Part model, mm, in its own coordinate system. Face numbers are marked on the shaded views. A direction names the side the tool comes from. Coordinates: 2 decimals unless noted, no trailing zeros. Loops run counter-clockwise (first coordinate to the right, second up) from the corner with the lowest first, then second, coordinate; pieces in that order, holes last. Notation, with made-up numbers: (-7.5, 31) -> (28.5, 31) arc R20 ccw to (28.5, 54) -> close; hole circle Ø10 at (-27, 83.5). An arc over 180 degrees is marked (long way). One line per question, with ' | ' between items. Start each with the question number.
1) Cut at C-C (y = 66.5). List the corners of the cut face in (x, z), plus the area to 3 significant figures.
2) Probe L1, parallel to X at y = 10, z = 38.5; L2, parallel to Y at x = 61, z = -28.5; L3, parallel to X at y = 67, z = -42.5. List the from-to ranges inside material, lowest first. Write a range as from..to.
3) 3-axis set-ups, long thin cutter, end or side, ignore diameter. For the marked faces 1 and 2: which of +Z, -Z, +X, -X, +Y, -Y reach the whole face in a straight line?
4) Drop flat-ended pins along their axis: pin 1 (1.2 mm diameter, centred on x = 79.45, z = -62.77, fed in from -Y); pin 2 (2 mm diameter, centred on x = 28, z = 47, fed in from -Y). Give the stop position or say it passes through.
5) Two-plate mould, pull along X, no slides. Class the marked faces 3, 4 and 5: released by +X, released by -X, zero draft, split by the parting line, or undercut.
6) Cut at A-A (y = 29.5). List the corners of the cut face in (x, z), plus the area to 3 significant figures.
7) Cut at B-B (z = -47). List the corners of the cut face in (x, y), plus the area to 4 significant figures.
8) Cut at D-D (x = 65). List the corners of the cut face in (y, z).
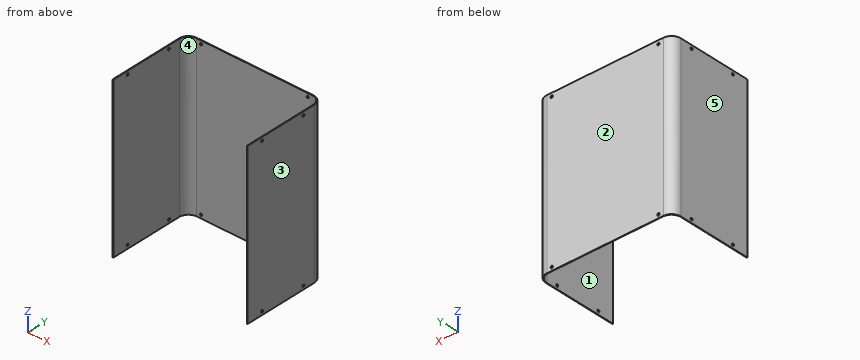
from build123d import *

# Parameters (mm, degrees)
SKETCH_1_W          = 117
SKETCH_1_H          = 138
EXTRUDE_1_DEPTH     = 72.5
CUT_EXTRUDE_1_DEPTH = 140
CUT_EXTRUDE_2_DEPTH = 140
SKETCH_6_R          = 1
CUT_EXTRUDE_5_DEPTH = 140
SKETCH_7_R          = 1
CUT_EXTRUDE_7_DEPTH = 140


with BuildPart() as part:
    # Эскиз1 → Бобышка-Вытянуть1 (new body)
    with BuildSketch(Plane(origin=(0, 0, 0), x_dir=(1, 0, 0), z_dir=(0, 1, 0))):
        with Locations((33.234281685, -3.234040823)):
            Rectangle(SKETCH_1_W, SKETCH_1_H)
    extrude(amount=EXTRUDE_1_DEPTH)

    # Эскиз2 → Вырез-Вытянуть1 (cut)
    with BuildSketch(Plane(origin=(0, 0, -65.765959177), x_dir=(-1, 0, 0), z_dir=(0, 0, -1))):
        with BuildLine():
            Line((-91.734281685, 64.5), (-91.734281685, 72.5))
            Line((-91.734281685, 72.5), (-83.734281685, 72.5))
            ThreePointArc((-83.734281685, 72.5), (-89.391135935, 70.156854249), (-91.734281685, 64.5))
        make_face()
        with BuildLine():
            Line((17.265718315, 72.5), (25.265718315, 72.5))
            Line((25.265718315, 72.5), (25.265718315, 64.5))
            ThreePointArc((25.265718315, 64.5), (22.922572564, 70.156854249), (17.265718315, 72.5))
        make_face()
    extrude(amount=-CUT_EXTRUDE_1_DEPTH, mode=Mode.SUBTRACT)

    # Эскиз3 → Вырез-Вытянуть2 (cut)
    with BuildSketch(Plane.XY.offset(72.234040823)):
        with BuildLine():
            Line((-24.765718315, 0), (91.234281685, 0))
            Line((91.234281685, 0), (91.234281685, 64))
            ThreePointArc((91.234281685, 64), (88.891135935, 69.656854249), (83.234281685, 72))
            Line((83.234281685, 72), (-16.765718315, 72))
            ThreePointArc((-16.765718315, 72), (-22.422572564, 69.656854249), (-24.765718315, 64))
            Line((-24.765718315, 64), (-24.765718315, 0))
        make_face()
    extrude(amount=-CUT_EXTRUDE_2_DEPTH, mode=Mode.SUBTRACT)

    # Эскиз6 → Вырез-Вытянуть5 (cut)
    with BuildSketch(Plane.ZY.offset(25.265718315)):
        with Locations((-62.765959177, 14)):
            Circle(SKETCH_6_R)
        with Locations(Location((69.234040823, 14, 0), (0, 0, 270))):
            Circle(SKETCH_6_R)
        with Locations((-62.765959177, 54)):
            Circle(SKETCH_6_R)
        with Locations(Location((69.234040823, 54, 0), (0, 0, 270))):
            Circle(SKETCH_6_R)
    extrude(amount=-CUT_EXTRUDE_5_DEPTH, mode=Mode.SUBTRACT)

    # Эскиз7 → Вырез-Вытянуть7 (cut)
    with BuildSketch(Plane(origin=(0, 72, 0), x_dir=(-1, 0, 0), z_dir=(0, -1, 0))):
        with Locations(Location((-79.454291209, 62.765959177, 0), (0, 0, 90))):
            Circle(SKETCH_7_R)
        with Locations((-582.904668668, 16.142688411)):
            Circle(SKETCH_7_R)
        with Locations(Location((12.9857274, -69.234040823, 0), (0, 0, 90))):
            Circle(SKETCH_7_R)
        with Locations(Location((-79.454291209, -69.234040823, 0), (0, 0, 90))):
            Circle(SKETCH_7_R)
        with Locations(Location((12.985727838, 62.765959177, 0), (0, 0, 90))):
            Circle(SKETCH_7_R)
    extrude(amount=-CUT_EXTRUDE_7_DEPTH, mode=Mode.SUBTRACT)


solid = part.part
Reported:
1) outline: (-25.01, -65.77) -> (-24.37, -65.77) -> (-24.37, 72.23) -> (-25.01, 72.23) -> close; (90.83, -65.77) -> (91.48, -65.77) -> (91.48, 72.23) -> (90.83, 72.23) -> close | area: 178 mm²
2) L1: x = -25.27..-24.77, 91.23..91.73 | L2: y = 72..72.5 | L3: x = -24.87..-24.18, 90.65..91.33
3) face 1: +Z, -Z, -Y | face 2: +Z, -Z, +X, -X, +Y
4) pin 1: passes through | pin 2: stops at y = 72
5) face 3: released by +X | face 4: undercut | face 5: released by -X
6) outline: (-25.27, -65.77) -> (-24.77, -65.77) -> (-24.77, 72.23) -> (-25.27, 72.23) -> close; (91.23, -65.77) -> (91.73, -65.77) -> (91.73, 72.23) -> (91.23, 72.23) -> close | area: 138 mm²
7) outline: (-25.27, 0) -> (-24.77, 0) -> (-24.77, 64) arc R8 cw to (-16.77, 72) -> (83.23, 72) arc R8 cw to (91.23, 64) -> (91.23, 0) -> (91.73, 0) -> (91.73, 64.5) arc R8 ccw to (83.73, 72.5) -> (-17.27, 72.5) arc R8 ccw to (-25.27, 64.5) -> close | area: 130.5 mm²
8) outline: (72, -65.77) -> (72.5, -65.77) -> (72.5, 72.23) -> (72, 72.23) -> close
